Solid Edge part; units mm, degrees
sketch "Sketch1" plane through (0, 0, 0) normal (0, -1, 0) x (1, 0, 0)
  arc A0 (385.0032, 73.0943) -> (389.5032, 77.5943) centre (385.0032, 77.5943) ccw
  line L0 (389.5032, 77.5943) -> (389.5032, 172.7943)
  arc A1 (389.5032, 172.7943) -> (385.0032, 177.2943) centre (385.0032, 172.7943) ccw
  line L1 (385.0032, 177.2943) -> (223.8032, 177.2943)
  arc A2 (223.8032, 177.2943) -> (219.3032, 172.7943) centre (223.8032, 172.7943) ccw
  line L2 (219.3032, 172.7943) -> (219.3032, 77.5943)
  arc A3 (219.3032, 77.5943) -> (223.8032, 73.0943) centre (223.8032, 77.5943) ccw
  line L3 (223.8032, 73.0943) -> (385.0032, 73.0943)
extrude "Protrusion1" add sketch "Sketch1" against normal blind 4.3
sketch "Sketch2" plane through (304.4032, 4.3, 125.1943) normal (0, 1, 0) x (-1, 0, 0)
  line L0 (55, 28.4) -> (-55, 28.4)
  line L1 (-55, 28.4) -> (-55, -36.6)
  line L2 (-55, -36.6) -> (55, -36.6)
  line L3 (55, -36.6) -> (55, 28.4)
extrude "ExtrudedProtrusion_2" add sketch "Sketch2" along normal blind 55
fillet "Round_1" radius 5 8 edges at (304.4032, 59.3, 153.5943) (304.4032, 59.3, 88.5943) (359.4032, 59.3, 121.0943) (249.4032, 59.3, 121.0943) (359.4032, 31.8, 153.5943) (359.4032, 31.8, 88.5943) (249.4032, 31.8, 153.5943) (249.4032, 31.8, 88.5943)
The model under review builds one solid part; all positions refer to its coordinate system, in mm. A direction names the side the tool comes from. Coordinates: 2 decimals unless noted, no trailing zeros. Loops run counter-clockwise (first coordinate to the right, second up) from the corner with the lowest first, then second, coordinate; pieces in that order, holes last. Notation, with made-up numbers: (66.5, 30) -> (71.5, 30) arc R26 cw to (71.5, 58) -> close; hole circle Ø3 at (60, 59.5). An arc over 180 degrees is marked (long way). Use a Markdown table: item, result. Add a question column.
1. Add section B-B on y = 51. Write out the cut boundary in (x, z).
2. To check wall thickness, follow line 1 (X direction, y = 18.5, z = 123); line 2 (Z direction, x = 306, y = 18.5); line 3 (Y direction, x = 360, z = 153). State the ranges of each line that lie inside material, in increasing order.
3. Add section A-A on x = 315. Write out the cut boundary in (y, z).
4. Machinability: for faces 1 (the face through (359.403, 29, 121)), 2 (the face through (357.98, 29.65, 90.1)), 3 (the face through (249.403, 29, 121)), 4 (the face through (250.83, 29.65, 152.09)), 5 (the face through (304, 29, 153.594)), which of the approach directions +Z, -Z, +X, -X, +Y, -Y give a long, thin tool a straight path to every point of the face, cutting with its end or side? Answer none if there is none.
5. Add section C-C on z = 126.5. Write out the cut boundary in (x, y).
6. Clearance check with flat-ended pins moving along their axes: pin 1 Ø10 at (x, z) = (304, 84.5) entering from +Y; pin 2 Ø4 at (x, z) = (246.5, 90) entering from +Y; pin 3 Ø1 at (x, y) = (317, 18.5) entering from -Z. State where each tip first meets the part, or that it passes through.
7. Add section D-D on x = 375.5. Write out the cut boundary in (y, z).
Returned:
| question | item | result |
|---|---|---|
| 1 | outline | (249.4, 93.59) arc R5 ccw to (254.4, 88.59) -> (354.4, 88.59) arc R5 ccw to (359.4, 93.59) -> (359.4, 148.59) arc R5 ccw to (354.4, 153.59) -> (254.4, 153.59) arc R5 ccw to (249.4, 148.59) -> close |
| 2 | line 1 | x = 249.4 to 359.4 |
| 2 | line 2 | z = 88.59 to 153.59 |
| 2 | line 3 | y = 0 to 4.3 |
| 3 | outline | (0, 73.09) -> (4.3, 73.09) -> (4.3, 88.59) -> (54.3, 88.59) arc R5 ccw to (59.3, 93.59) -> (59.3, 148.59) arc R5 ccw to (54.3, 153.59) -> (4.3, 153.59) -> (4.3, 177.29) -> (0, 177.29) -> close |
| 4 | face 1 | +Z, -Z, +X, +Y |
| 4 | face 2 | -Z, +X, +Y |
| 4 | face 3 | +Z, -Z, -X, +Y |
| 4 | face 4 | +Z, -X, +Y |
| 4 | face 5 | +Z, +X, -X, +Y |
| 5 | outline | (219.3, 0) -> (389.5, 0) -> (389.5, 4.3) -> (359.4, 4.3) -> (359.4, 54.3) arc R5 ccw to (354.4, 59.3) -> (254.4, 59.3) arc R5 ccw to (249.4, 54.3) -> (249.4, 4.3) -> (219.3, 4.3) -> close |
| 6 | pin 1 | stops at y = 57.17 |
| 6 | pin 2 | stops at y = 4.3 |
| 6 | pin 3 | stops at z = 88.59 |
| 7 | outline | (0, 73.09) -> (4.3, 73.09) -> (4.3, 177.29) -> (0, 177.29) -> close |
